The figure shows three views and two pictorial views of one solid part (mm, origin at its lowest corner). Answer the questions. A direction names the side the tool comes from. Round coordinates to 2 decimals unless told otherwise and drop trailing zeros. Order: outer loops, then holes, each group sorted by start corner. A loop starts at its lowest first (then second) coordinate and runs counter-clockwise, first axis right, second up. Notation, with made-up numbers: M -16,3.5 L 26,3.5 A8 ccw 26,8.5 Z; hole C 58.5,-1.5 d2. An arc over 180 degrees is marked long. Answer as CSV lines item,"result".
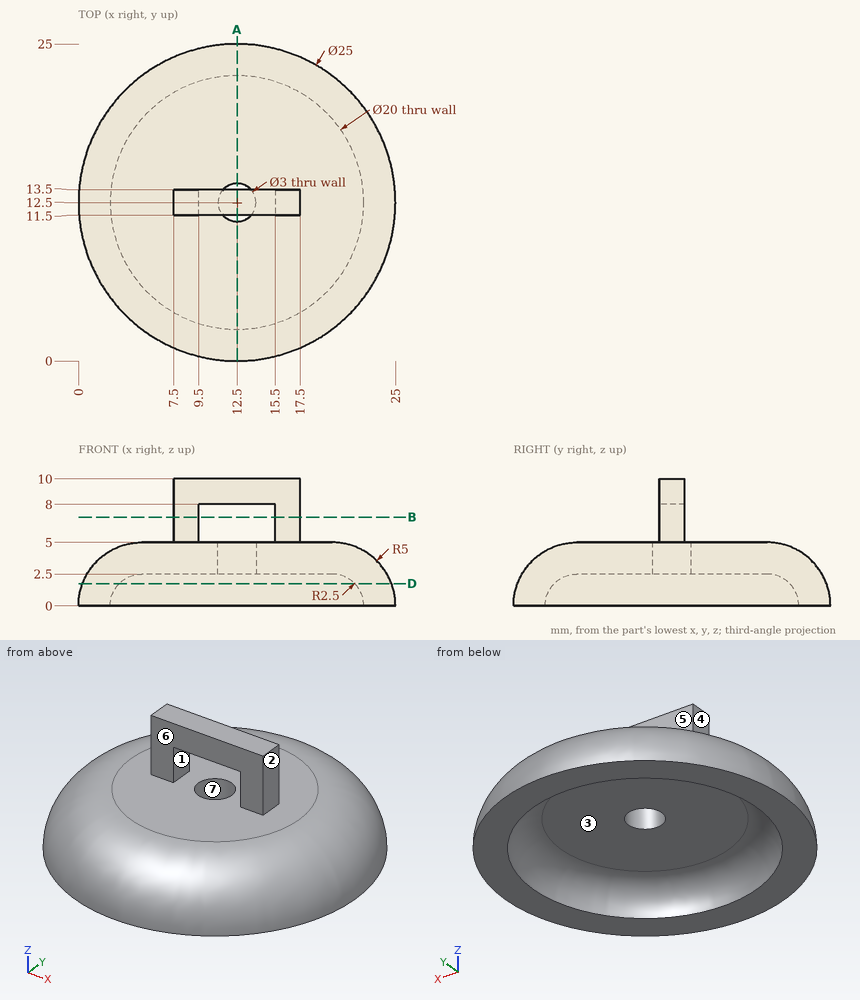
Item 1: Find the intervals of material crossed by probe 1 along Z at (x, y) = (11, 18.75); probe 2 along Y at (x, z) = (12.5, 0.05); probe 3 along X at (y, z) = (7.25, 1.25), in increasing order. Write a range as [from, to].
Ans:
probe 1,"[2.5, 5]"
probe 2,"[0, 2.5], [22.5, 25]"
probe 3,"[1.33, 4.39], [20.61, 23.67]"
Item 2: Determine the mould class of the marked faces 1, 2, 3 and 4 for opening direction X: +X half, -X half, draft (parallel to the pull), parting line (faces both ways), or undercut.
Ans:
face 1,"undercut"
face 2,"+X half"
face 3,"undercut"
face 4,"-X half"
Item 3: A cutting plane is placed at B-B, the plane z = 7. Determine the outline of the cut face in (x, y), and give its area (3 significant figures).
Ans:
outline,"M 7.5,11.5 L 9.5,11.5 L 9.5,13.5 L 7.5,13.5 Z; M 15.5,11.5 L 17.5,11.5 L 17.5,13.5 L 15.5,13.5 Z"
area,"8.00 mm2"
Item 4: A cutting plane is placed at A-A, the plane x = 12.5. Give the number of separate pieces and of enclosed holes in the cut face, and give its area (3 significant figures).
Ans:
separate pieces,"3"
enclosed holes,"0"
area,"63.5 mm2"
Item 5: A cutting plane is placed at D-D, the plane z = 1.75. Determine the outline of the cut face in (x, y), and give its area (3 significant figures).
Ans:
outline,"C 12.5,12.5 d24.37; hole C 12.5,12.5 d18.57"
area,"195 mm2"
Item 6: A tool of negligible diameter and unlimited length cuts with its end or side. For the marked faces 5, 6 and 7, from which of +Z, -Z, +X, -X, +Y, -Y can it reach the whole face along a straight path? Write none if from no direction.
Ans:
face 5,"+Z, +X, -X, +Y"
face 6,"+Z, +X, -X, -Y"
face 7,"-Z"
Item 7: Flat-ended cylindrical pins translate along their axes: pin 1 (3.5 mm diameter, centred on x = 12.5, y = 12.5, fed in from -Z); pin 2 (7.5 mm diameter, centred on x = 16, y = 9, fed in from -Z); pin 3 (2.5 mm diameter, centred on x = 13.5, z = 8.5, fed in from +Y). Find the tip coordinate at first contact, or state that the pin passes through.
Ans:
pin 1,"z = 2.5"
pin 2,"z = 2.19"
pin 3,"y = 13.5"
